Read the model definition and answer for the solid it produces. Units are mm, in the model's axes. A direction names the side the tool comes from. Coordinates: 2 decimals unless noted, no trailing zeros. Write each loop counter-clockwise with the first axis right and the second up, starting at its lowest first coordinate (ties: lowest second). Pieces come first, ordered by that corner, then holes.
1) Find the intervals of material crossed by line 1 (Y direction, x = -21.5, z = 1.1); line 2 (X direction, y = 5.25, z = 1.05); line 3 (X direction, y = 1.25, z = 1.45), in increasing order.
2) Determine the mould class of faces 4 (the face through (-26.49, 0.62, 0.99)), 5 (the face through (22, 0, 2)), 6 (the face through (-26.49, -0.01, 0.38)) for opening direction Z: +Z half, -Z half, draft (parallel to the pull), parting line (faces both ways), or undercut.
3) The part is cut by section B-B (y = -5). Determine the outline of the cut face in (x, z).
4) Which of the six approach directions +Z, -Z, +X, -X, +Y, -Y give full straight-line access (tool end or side, diameter ignored) to faces 1 (the face through (1, -1, 1)), 2 (the face through (40, 0, 1)), 3 (the face through (1, 1, 1))?
5) The part is cut by section A-A (x = -15). Determine the outline of the cut face in (y, z).
from build123d import *

# Parameters (mm, degrees)
SKETCH1_W           = 60
SKETCH1_H           = 2
BOSS_EXTRUDE1_DEPTH = 2
CHAMFER1_SIZE       = 5.67128182
CHAMFER1_SIZE_2     = 1
FILLET1_R           = 5
FILLET2_R           = 3


# Some blends are built 0.0001 mm under size
with BuildPart() as part:
    # Sketch1 → Boss-Extrude1 (new body)
    with BuildSketch(Plane.XY):
        Rectangle(SKETCH1_W, SKETCH1_H)
        Polygon((30, 1), (30, -1), (30, -7.5), (40, -7.5), (40, 7.5), (30, 7.5), align=None)
    extrude(amount=BOSS_EXTRUDE1_DEPTH)

    # Chamfer1
    # the kernel refuses this chamfer: 5.67128182, 1 mm, written as the material it takes off along each edge
    with BuildSketch(Plane(origin=(-30, -15.737045834, 0), x_dir=(0.9999776716360547, 0, -0.006682531656101592), z_dir=(0, 1, 0)), Plane(origin=(-30, 1, -14.737045834), x_dir=(0.9999776716360547, 0.00668253165610172, 0), z_dir=(0, 0, 1))) as chamfer1_piece_1:
        Polygon((CHAMFER1_SIZE * 0.999977671569, -CHAMFER1_SIZE * 0.00668253165565), (-CHAMFER1_SIZE_2 * 0.00668253165611, -CHAMFER1_SIZE_2 * 0.999977671636), (0, 0), align=None)
    extrude(amount=31.474091667, mode=Mode.SUBTRACT)
    with BuildSketch(Plane(origin=(-30, -1, -14.737045834), x_dir=(-0.21013876076743543, 0.9776715712462578, 0), z_dir=(0, 0, 1))) as chamfer1_piece_2:
        Polygon((CHAMFER1_SIZE_2 * 0.977671571246, -CHAMFER1_SIZE_2 * 0.210138760767), (-CHAMFER1_SIZE * 0.210138760753, -CHAMFER1_SIZE * 0.97767157118), (0, 0), align=None)
    extrude(amount=31.474091667, mode=Mode.SUBTRACT)
    with BuildSketch(Plane(origin=(-30, -15.737045834, 2), x_dir=(0.9999776716360547, 0, 0.006682531656101588), z_dir=(0, 1, 0))) as chamfer1_piece_3:
        Polygon((CHAMFER1_SIZE * 0.999977671569, CHAMFER1_SIZE * 0.00668253165565), (-CHAMFER1_SIZE_2 * 0.00668253165611, CHAMFER1_SIZE_2 * 0.999977671636), (0, 0), align=None)
    extrude(amount=31.474091667, mode=Mode.SUBTRACT)

    # Fillet1
    fillet1_edges = [part.edges().sort_by_distance(p)[0] for p in [
        (40, -7.5, 1),
        (40, 7.5, 1),
        (30, 7.5, 1),
        (30, -7.5, 1),
    ]]
    fillet(fillet1_edges, radius=FILLET1_R - 0.0001)  # a hair under: the kernel refuses the full size

    # Fillet2
    fillet2_edges = [part.edges().sort_by_distance(p)[0] for p in [
        (30, 1, 1),
        (30, -1, 1),
    ]]
    fillet(fillet2_edges, radius=FILLET2_R)


solid = part.part
Reported:
1. line 1: y = -1 to 1
1. line 2: x = 30.82 to 39.18
1. line 3: x = 28.34 to 40
2. face 4: draft
2. face 5: +Z half
2. face 6: -Z half
3. outline: (30.67, 0) - (39.33, 0) - (39.33, 2) - (30.67, 2) - close
4. face 1: +Z, -Z, -X, -Y
4. face 2: +Z, -Z, +X, +Y, -Y
4. face 3: +Z, -Z, -X, +Y
5. outline: (-1, 0) - (1, 0) - (1, 2) - (-1, 2) - close
